Part model, mm, in its own coordinate system. Face numbers are marked on the shaded views. A direction names the side the tool comes from. Coordinates: 2 decimals unless noted, no trailing zeros. Loops run counter-clockwise (first coordinate to the right, second up) from the corner with the lowest first, then second, coordinate; pieces in that order, holes last.
```python
from build123d import *

# Parameters (mm, degrees)
F0_W     = 1.5875
F0_H     = 1.5875
F3_DEPTH = 1.5875
F4_R     = 3.175
F4_R_2   = 2.38125
F5_DEPTH = 1.5875


with BuildPart() as f1:
    # F0 (on Front) → F1 (revolve)
    with BuildSketch(Plane.XZ):
        with Locations((11.1125, 0.79375)):
            Rectangle(F0_W, F0_H)
        Polygon((0, 19.05), (0, 1.5875), (10.31875, 1.5875), (11.90625, 1.5875), (7.9375, 19.05), align=None)
    revolve(axis=Axis((0, 0, 9.525), (0, 0, 1)))

    # F2 (on face) → F3 (join)
    with BuildSketch(Plane.XY.offset(19.05)):
        with BuildLine():
            ThreePointArc((6.028877012, 5.162997988), (5.6126600757, 5.6126600757), (5.162997988, 6.028877012))
            ThreePointArc((5.162997988, 6.028877012), (1.9054814058, 2.7799378741), (6.35, 3.96875))
            ThreePointArc((6.35, 3.96875), (6.2683183301, 4.5870840986), (6.028877012, 5.162997988))
        make_face()
        with BuildLine():
            ThreePointArc((-1.5875, 3.96875), (-2.7799378741, 6.0320185942), (-5.162997988, 6.028877012))
            ThreePointArc((-5.162997988, 6.028877012), (-5.6126600757, 5.6126600757), (-6.028877012, 5.162997988))
            ThreePointArc((-6.028877012, 5.162997988), (-4.5870840986, 1.6691816699), (-1.5875, 3.96875))
        make_face()
        with BuildLine():
            ThreePointArc((-6.028877012, -5.162997988), (-5.6126600757, -5.6126600757), (-5.162997988, -6.028877012))
            ThreePointArc((-5.162997988, -6.028877012), (-2.7799378741, -6.0320185942), (-1.5875, -3.96875))
            ThreePointArc((-1.5875, -3.96875), (-4.5870840986, -1.6691816699), (-6.028877012, -5.162997988))
        make_face()
        with BuildLine():
            ThreePointArc((6.35, -3.96875), (1.9054814058, -2.7799378741), (5.162997988, -6.028877012))
            ThreePointArc((5.162997988, -6.028877012), (5.6126600757, -5.6126600757), (6.028877012, -5.162997988))
            ThreePointArc((6.028877012, -5.162997988), (6.2683183301, -4.5870840986), (6.35, -3.96875))
        make_face()
    extrude(amount=F3_DEPTH)

    # F4 (on face) → F5 (join)
    with BuildSketch(Plane(origin=(0, 0, 1.5875), x_dir=(1, 0, 0), z_dir=(0, 0, -1))):
        with Locations((-4.7625, -4.7625)):
            Circle(F4_R)
        with Locations((-4.7625, -4.7625)):
            Circle(F4_R_2, mode=Mode.SUBTRACT)
        with Locations((-4.7625, 4.7625)):
            Circle(F4_R)
        with Locations((-4.7625, 4.7625)):
            Circle(F4_R_2, mode=Mode.SUBTRACT)
        with Locations((4.7625, -4.7625)):
            Circle(F4_R)
        with Locations((4.7625, -4.7625)):
            Circle(F4_R_2, mode=Mode.SUBTRACT)
        with Locations((4.7625, 4.7625)):
            Circle(F4_R)
        with Locations((4.7625, 4.7625)):
            Circle(F4_R_2, mode=Mode.SUBTRACT)
    extrude(amount=F5_DEPTH)


solid = f1.part
```
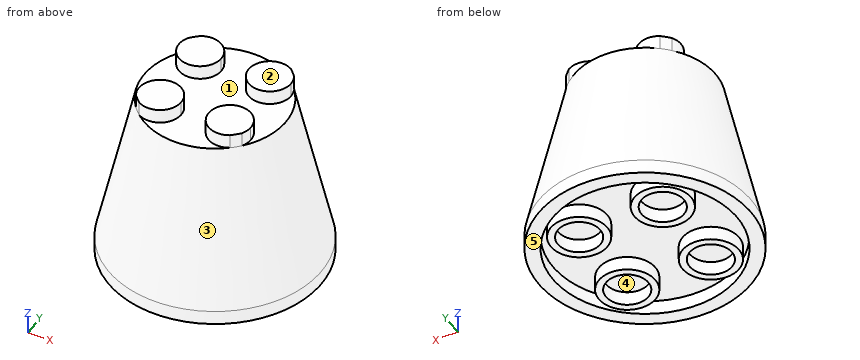
Q1. Mould opens along Y. For the marked faces 1, 2 and 3 say: released by +Y, released by -Y, zero draft, split by the parting line, or undercut.
Q2. Saw through at D-D (z = 9.25). List the corners of the cut face in (x, y), plus the area to 3 significant figures.
Q3. Saw through at A-A (z = 19.5). Count the separate pieces of the cut face and the enclosed holes in it, plus the area to 3 significant figures.
Q4. Tool access for the marked faces 4 and 5: list every direction of +Z, -Z, +X, -X, +Y, -Y with a clear straight run to the whole face (end or side of a thin tool).
Q5. Drop flat-ended pins along their axis: P1, Ø10, axis at x = 6.5, z = 5, coming from the -Y side; P2, Ø5, axis at y = 7.5, z = 2.5, coming from the +X side; P3, Ø6, axis at x = -7, z = 7.5, coming from the +Y side. Give the stop position or say it passes through.
Q6. Probe line 1 (Y direction, x = 0, z = 1.2); line 2 (Z direction, x = -1.25, y = -0.5); line 3 (Z direction, x = 2.25, y = 5.75). List the from-to ranges inside material, lowest first.
Q7. Saw through at B-B (y = 0). List the corners of the cut face in (x, z), plus the area to 3 significant figures.
Checked values:
1. face 1: undercut
1. face 2: zero draft
1. face 3: split by the parting line
2. outline: circle Ø20.33 at (0, 0)
2. area: 325 mm2
3. separate pieces: 4
3. enclosed holes: 0
3. area: 71.1 mm2
4. face 4: -Z
4. face 5: -Z, +X, -X, +Y, -Y
5. P1: stops at y = -11.56
5. P2: stops at x = 10.72
5. P3: stops at y = 9.98
6. line 1: y = -11.91 to -10.32, 10.32 to 11.91
6. line 2: z = 1.59 to 19.05
6. line 3: z = 0 to 19.05
7. outline: (-11.91, 0) - (-10.32, 0) - (-10.32, 1.59) - (10.32, 1.59) - (10.32, 0) - (11.91, 0) - (11.91, 1.59) - (7.94, 19.05) - (-7.94, 19.05) - (-11.91, 1.59) - close
7. area: 352 mm2
